```python
from build123d import *

# Parameters (mm, degrees)
SKETCH_R           = 2.95
PAD_DEPTH          = 8.5
SKETCH001_R        = 4.5
PAD001_DEPTH       = 0.5
SKETCH002_R        = 7.5
PAD002_DEPTH       = 3
SKETCH003_R        = 1.25
HOLE_DEPTH         = 12.001
POCKET_DEPTH       = 60.74523
POLARPATTERN_COUNT = 50


with BuildPart() as part:
    # Sketch → Pad (new body)
    with BuildSketch(Plane.XY):
        Circle(SKETCH_R)
    extrude(amount=PAD_DEPTH)

    # Sketch001 (on Face4 of Pad) → Pad001 (join)
    with BuildSketch(Plane.XY.offset(8.5)):
        Circle(SKETCH001_R)
    extrude(amount=PAD001_DEPTH)

    # Sketch002 (on Face7 of Pad001) → Pad002 (join)
    with BuildSketch(Plane.XY.offset(9)):
        Circle(SKETCH002_R)
    extrude(amount=PAD002_DEPTH)

    # Sketch003 (on Face7 of Pad002) → Hole (cut, through all)
    with BuildSketch(Plane.XY.offset(12)):
        Circle(SKETCH003_R)
    extrude(amount=-HOLE_DEPTH, mode=Mode.SUBTRACT)

    # Sketch004 (on Face5 of Hole) → Pocket (cut, through all)
    with BuildSketch(Plane.XY.offset(12)):
        Polygon((7.1, 0), (7.533013, 0.25), (7.533013, -0.25), align=None)
    pocket = extrude(amount=-POCKET_DEPTH, mode=Mode.SUBTRACT)

    # PolarPattern: Pocket ×50 about axis
    polarpattern_axis = Axis((0, 0, 12), (0, 0, 1))
    for i in range(1, POLARPATTERN_COUNT):
        add(pocket.rotate(polarpattern_axis, i * 360 / POLARPATTERN_COUNT), mode=Mode.SUBTRACT)


solid = part.part
```
Build history of the part. All positions in model axes, mm. A direction names the side the tool comes from. Give positions to 0.01 mm unless a question says otherwise; leave off trailing zeros. Loops run counter-clockwise (first coordinate to the right, second up) from the corner with the lowest first, then second, coordinate; pieces in that order, holes last. Notation, with made-up numbers: (88.5, 43.5) - (137.5, 43.5) arc R19 cw to (137.5, 79.5) - close; hole circle Ø2 at (-1.75, 83). An arc over 180 degrees is marked (long way). Use a Markdown table: item, result.
(1) Pull direction Y, two halves, no side cores. Call faces 1 (the face through (-2.947, 0.13, 4.19)), 2 (the face through (1, -3, 8.5)), 3 (the face through (-0.27, -1.22, 6.08)): +Y half, -Y half, draft (parallel to the pull), parting line (faces both ways), or undercut.
Taken from the geometry:
| item | result |
|---|---|
| face 1 | parting line |
| face 2 | draft |
| face 3 | undercut |
(2) Drop flat-ended pins along their axis: pin 1 Ø5 at (y, z) = (-5, 3) entering from -X; pin 2 Ø3 at (x, z) = (-4, 6) entering from +Y; pin 3 Ø1 at (y, z) = (-2, 1.5) entering from +X; pin 4 Ø2 at (x, y) = (0, 0) entering from +Z. Give the stop position or say it passes through.
Taken from the geometry:
| item | result |
|---|---|
| pin 1 | x = -1.57 |
| pin 2 | y = 1.57 |
| pin 3 | x = 2.54 |
| pin 4 | through |
(3) Which spindle directions (+Z, -Z, +X, -X, +Y, -Y) get a long thin tool onto all of the face, cutting with end or side? Do faces 4 (the face through (-0.59, 4.46, 8.75)), 5 (the face through (1, -1, 0)). Say none if no direction does.
Taken from the geometry:
| item | result |
|---|---|
| face 4 | -Z |
| face 5 | -Z, +X, -X, +Y, -Y |
(4) Band-saw the part on B-B (z = 7.5). Give the cut face in (x, y), and give its area (3 significant figures).
Taken from the geometry:
| item | result |
|---|---|
| outline | circle Ø5.9 at (0, 0); hole circle Ø2.5 at (0, 0) |
| area | 22.4 mm2 |
(5) Wall check: line 1 along Y through (x, z) = (0, 5); line 2 along Y through (x, z) = (0, 8.75); line 3 along Z through (x, y) = (5.5, -3). Give the ranges that are in metal, low to high.
Taken from the geometry:
| item | result |
|---|---|
| line 1 | -2.95 to -1.25, 1.25 to 2.95 |
| line 2 | -4.5 to -1.25, 1.25 to 4.5 |
| line 3 | 9 to 12 |
(6) Band-saw the part on C-C (x = 2.75). Give the cut face in (y, z), and give its area (3 significant figures).
Taken from the geometry:
| item | result |
|---|---|
| outline | (-6.98, 9) - (-3.56, 9) - (-3.56, 8.5) - (-1.07, 8.5) - (-1.07, 0) - (1.07, 0) - (1.07, 8.5) - (3.56, 8.5) - (3.56, 9) - (6.98, 9) - (6.98, 12) - (-6.98, 12) - close |
| area | 63.6 mm2 |
(7) Band-saw the part on A-A (x = 0). Give the cut face in (y, z).
Taken from the geometry:
| item | result |
|---|---|
| outline | (-7.5, 9) - (-4.5, 9) - (-4.5, 8.5) - (-2.95, 8.5) - (-2.95, 0) - (-1.25, 0) - (-1.25, 12) - (-7.5, 12) - close; (1.25, 0) - (2.95, 0) - (2.95, 8.5) - (4.5, 8.5) - (4.5, 9) - (7.5, 9) - (7.5, 12) - (1.25, 12) - close |
